```python
from build123d import *

# Parameters (mm, degrees)
F0_R     = 1.5939084554
F1_DEPTH = 3.048


with BuildPart() as f1:
    # F0 (on Front) → F1 (new body)
    with BuildSketch(Plane.XZ):
        with BuildLine():
            ThreePointArc((-37.513228268, 58.1266457065), (-37.5049761739, 58.3554311802), (-37.5022249461, 58.5843488964))
            ThreePointArc((-37.5022249461, 58.5843488964), (-37.6124710423, 60.0293519865), (-37.9406572675, 61.4409050085))
            Line((-37.9406572675, 61.4409050085), (-37.513228268, 58.1266457065))
        make_face()
        with BuildLine():
            Line((-37.513228268, 58.1266457065), (-37.9406572675, 61.4409050085))
            ThreePointArc((-37.9406572675, 61.4409050085), (-47.3561500663, 68.1036678461), (-56.2892930862, 60.8068967067))
            Line((-56.2892930862, 60.8068967067), (-56.5510749385, 58.7323567411))
            ThreePointArc((-56.5510749385, 58.7323567411), (-53.8145439942, 51.9016903581), (-47.0272249461, 49.0593488964))
            ThreePointArc((-47.0272249461, 49.0593488964), (-40.4558475366, 51.689232948), (-37.513228268, 58.1266457065))
        make_face()
        with BuildLine():
            ThreePointArc((-43.8522249461, 58.5843488964), (-44.7821609158, 56.3392848661), (-47.0272249461, 55.4093488964))
            ThreePointArc((-47.0272249461, 55.4093488964), (-49.2722889764, 60.8294129267), (-43.8522249461, 58.5843488964))
        make_face(mode=Mode.SUBTRACT)
        with BuildLine():
            Line((-31.2826202902, 9.8148781945), (-37.513228268, 58.1266457065))
            ThreePointArc((-37.513228268, 58.1266457065), (-40.4558475366, 51.689232948), (-47.0272249461, 49.0593488964))
            Line((-47.0272249461, 49.0593488964), (-47.0272249461, 23.6593488964))
            ThreePointArc((-47.0272249461, 23.6593488964), (-36.5443586302, 19.7059737355), (-31.2826202902, 9.8148781945))
        make_face()
        with BuildLine():
            Line((-56.5510749385, 58.7323567411), (-56.2892930862, 60.8068967067))
            ThreePointArc((-56.2892930862, 60.8068967067), (-56.4772836251, 59.7768320044), (-56.5510749385, 58.7323567411))
        make_face()
        with BuildLine():
            Line((-47.0272249461, 23.6593488964), (-47.0272249461, 49.0593488964))
            ThreePointArc((-47.0272249461, 49.0593488964), (-53.8145439942, 51.9016903581), (-56.5510749385, 58.7323567411))
            Line((-56.5510749385, 58.7323567411), (-62.5761934224, 10.9851619686))
            ThreePointArc((-62.5761934224, 10.9851619686), (-57.0572478145, 20.0893993335), (-47.0272249461, 23.6593488964))
        make_face()
        with Locations((-49.5402999222, 46.5105995536)):
            Circle(F0_R, mode=Mode.SUBTRACT)
        with BuildLine():
            ThreePointArc((-31.1522249461, 7.7843488964), (-31.1848573214, 8.8017048047), (-31.2826202902, 9.8148781945))
            ThreePointArc((-31.2826202902, 9.8148781945), (-36.5443586302, 19.7059737355), (-47.0272249461, 23.6593488964))
            Line((-47.0272249461, 23.6593488964), (-47.0272249461, 10.9593488964))
            ThreePointArc((-47.0272249461, 10.9593488964), (-44.7821609158, 10.0294129267), (-43.8522249461, 7.7843488964))
            ThreePointArc((-43.8522249461, 7.7843488964), (-44.7821609158, 5.5392848661), (-47.0272249461, 4.6093488964))
            Line((-47.0272249461, 4.6093488964), (-47.0272249461, -8.0906511036))
            ThreePointArc((-47.0272249461, -8.0906511036), (-36.9406754756, -4.4744089844), (-31.4494526235, 4.7267952233))
            Line((-31.4494526235, 4.7267952233), (-31.1523694634, 7.7166111531))
            ThreePointArc((-31.1523694634, 7.7166111531), (-31.1522610755, 7.7504799477), (-31.1522249461, 7.7843488964))
        make_face()
        with BuildLine():
            Line((-47.0272249461, 10.9593488964), (-47.0272249461, 23.6593488964))
            ThreePointArc((-47.0272249461, 23.6593488964), (-57.0572478145, 20.0893993335), (-62.5761934224, 10.9851619686))
            ThreePointArc((-62.5761934224, 10.9851619686), (-62.849805464, 9.0733681958), (-62.8892440844, 7.1424970002))
            Line((-62.8892440844, 7.1424970002), (-62.7019557202, 5.2706981331))
            ThreePointArc((-62.7019557202, 5.2706981331), (-57.3255602274, -4.2970382521), (-47.0272249461, -8.0906511036))
            Line((-47.0272249461, -8.0906511036), (-47.0272249461, 4.6093488964))
            ThreePointArc((-47.0272249461, 4.6093488964), (-50.2022249461, 7.7843488964), (-47.0272249461, 10.9593488964))
        make_face()
        with BuildLine():
            ThreePointArc((-31.4494526235, 4.7267952233), (-31.2300195353, 6.2146590511), (-31.1523694634, 7.7166111531))
            Line((-31.1523694634, 7.7166111531), (-31.4494526235, 4.7267952233))
        make_face()
        with BuildLine():
            Line((-62.7019557202, 5.2706981331), (-62.8892440844, 7.1424970002))
            ThreePointArc((-62.8892440844, 7.1424970002), (-62.8233496768, 6.203820981), (-62.7019557202, 5.2706981331))
        make_face()
        with BuildLine():
            Line((-35.7167991292, -38.2193635433), (-31.4494526235, 4.7267952233))
            ThreePointArc((-31.4494526235, 4.7267952233), (-36.9406754756, -4.4744089844), (-47.0272249461, -8.0906511036))
            Line((-47.0272249461, -8.0906511036), (-47.0272249461, -46.1906511036))
            ThreePointArc((-47.0272249461, -46.1906511036), (-40.2920328553, -48.9804590128), (-37.5022249461, -55.7156511036))
            Line((-37.5022249461, -55.7156511036), (-15.310948927, -55.7156511036))
            ThreePointArc((-15.310948927, -55.7156511036), (-12.8738194092, -49.9929043149), (-7.0590230542, -47.7843811788))
            Line((-7.0590230542, -47.7843811788), (-28.1204876136, -46.9494241745))
            ThreePointArc((-28.1204876136, -46.9494241745), (-33.8031377964, -44.2241541431), (-35.7167991292, -38.2193635433))
        make_face()
        with BuildLine():
            ThreePointArc((-47.0272249461, -8.0906511036), (-57.3255602274, -4.2970382521), (-62.7019557202, 5.2706981331))
            Line((-62.7019557202, 5.2706981331), (-56.5048997845, -56.6639678528))
            ThreePointArc((-56.5048997845, -56.6639678528), (-54.0897436907, -49.3245280425), (-47.0272249461, -46.1906511036))
            Line((-47.0272249461, -46.1906511036), (-47.0272249461, -8.0906511036))
        make_face()
        with BuildLine():
            ThreePointArc((-47.0272249461, -46.1906511036), (-54.0897436907, -49.3245280425), (-56.5048997845, -56.6639678528))
            ThreePointArc((-56.5048997845, -56.6639678528), (-53.0237393117, -63.1161538205), (-45.9900241775, -65.1840110231))
            ThreePointArc((-45.9900241775, -65.1840110231), (-39.9348007371, -62.0735708766), (-37.5022249461, -55.7156511036))
            Line((-37.5022249461, -55.7156511036), (-43.8522249461, -55.7156511036))
            ThreePointArc((-43.8522249461, -55.7156511036), (-49.2722889764, -57.9607151339), (-47.0272249461, -52.5406511036))
            Line((-47.0272249461, -52.5406511036), (-47.0272249461, -46.1906511036))
        make_face()
        with BuildLine():
            ThreePointArc((-37.5022249461, -55.7156511036), (-39.9348007371, -62.0735708766), (-45.9900241775, -65.1840110231))
            Line((-45.9900241775, -65.1840110231), (-7.0603012501, -63.6469715978))
            ThreePointArc((-7.0603012501, -63.6469715978), (-12.8742805261, -61.4379546579), (-15.310948927, -55.7156511036))
            Line((-15.310948927, -55.7156511036), (-37.5022249461, -55.7156511036))
        make_face()
        with BuildLine():
            ThreePointArc((0.564051073, -55.7156511036), (-1.6507021383, -50.2152806213), (-7.0590230542, -47.7843811788))
            ThreePointArc((-7.0590230542, -47.7843811788), (-12.8738194092, -49.9929043149), (-15.310948927, -55.7156511036))
            ThreePointArc((-15.310948927, -55.7156511036), (-12.8742805261, -61.4379546579), (-7.0603012501, -63.6469715978))
            ThreePointArc((-7.0603012501, -63.6469715978), (-1.6511453727, -61.2164827028), (0.564051073, -55.7156511036))
        make_face()
        with BuildLine():
            ThreePointArc((-4.198448927, -55.7156511036), (-7.373448927, -58.8906511036), (-10.548448927, -55.7156511036))
            ThreePointArc((-10.548448927, -55.7156511036), (-7.373448927, -52.5406511036), (-4.198448927, -55.7156511036))
        make_face(mode=Mode.SUBTRACT)
        with BuildLine():
            ThreePointArc((-37.5022249461, -55.7156511036), (-40.2920328553, -48.9804590128), (-47.0272249461, -46.1906511036))
            Line((-47.0272249461, -46.1906511036), (-47.0272249461, -52.5406511036))
            ThreePointArc((-47.0272249461, -52.5406511036), (-44.7821609158, -53.4705870733), (-43.8522249461, -55.7156511036))
            Line((-43.8522249461, -55.7156511036), (-37.5022249461, -55.7156511036))
        make_face()
    extrude(amount=F1_DEPTH)


solid = f1.part
```
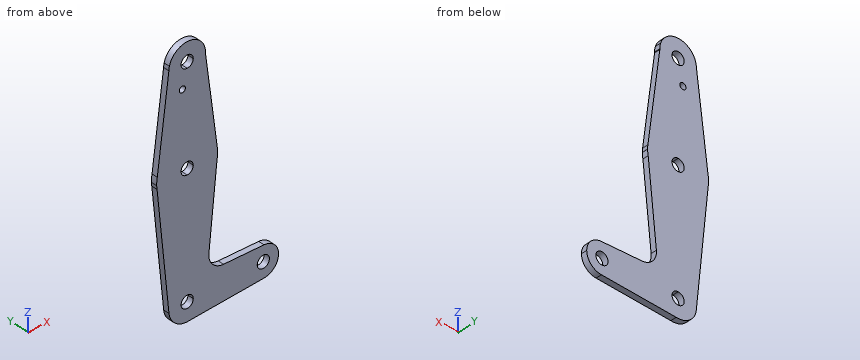
Input: part model. Units: mm. Frame: model coordinates. Coordinates: 2 decimals unless noted, no trailing zeros. Loops run counter-clockwise (first coordinate to the right, second up) from the corner with the lowest first, then second, coordinate; pieces in that order, holes last. Notation, with made-up numbers: M -34.5,-0.5 L -27.5,-0.5 A7 ccw -27.5,3.5 Z; hole C -8.75,-25.75 d3. An arc over 180 degrees is marked long. Use a Markdown table: item, result. Add a question column.
1) Section C-C, the plane z = -16. Return the cut outline in (x, y).
2) Section A-A, the plane y = -1.6. Give the number of separate pieces and of enclosed holes in the cut face, plus the area to 3 significant figures.
3) Section B-B, the plane x = -53. Return the cut outline in (y, z).
4) Pin query (flat end, axial travel): P1, Ø1.5, axis at x = -43, y = -1, coming from the -Z side; P2, Ø4, axis at x = -47.03, z = 58.58, coming from the +Y side; P3, Ø1.5, axis at y = -2, z = 41.5, coming from the -X side; P4, Ø12, axis at x = -31.5, z = -28.5, coming from the +Y side. Return the tip coordinate at first contact, or that it passes through.
5) Line query: L1, parallel to X at y = -2.8, z = -55; L2, parallel to X at y = -2, z = 11; L3, parallel to Z at x = -4.5, y = -2.1. Output: solid intervals per line, ascending. Write a range as from..to.
Answer below:
| question | item | result |
|---|---|---|
| 1 | outline | M -60.57,-3.05 L -33.51,-3.05 L -33.51,0 L -60.57,0 Z |
| 2 | separate pieces | 1 |
| 2 | enclosed holes | 5 |
| 2 | area | 3,700 mm2 |
| 3 | outline | M -3.05,-63.14 L 0,-63.14 L 0,66 L -3.05,66 Z |
| 4 | P1 | z = -65.1 |
| 4 | P2 | through |
| 4 | P3 | x = -58.82 |
| 4 | P4 | y = 0 |
| 5 | L1 | -56.67..-50.12, -43.93..-10.47, -4.28..0.53 |
| 5 | L2 | -62.57..-31.44 |
| 5 | L3 | -63.11..-57.07, -54.37..-48.32 |
